Can you work these out from the model? Positions are in its coordinate system, mm. A direction names the side the tool comes from. Round coordinates to 2 decimals unless told otherwise and drop trailing zeros. Write each loop counter-clockwise with the first axis right and the second up, starting at its lowest first coordinate (ties: lowest second). Pieces come first, ordered by that corner, then holes. Notation, with made-up numbers: M 4,14 L 45,14 A4 ccw 45,19 Z; hole C -6,28.5 d4. An arc over 180 degrees is marked long. Answer as a JSON object with one key per item and string values. Group by question number.
1) I'm going to push flat-ended pins straight in: pin 1 Ø23 at (x, z) = (25.4, -25.4) entering from +Y; pin 2 Ø3 at (x, y) = (13, 72.5) entering from -Z; pin 3 Ø3 at (x, y) = (34.5, 38.5) entering from +Z. Where does each tip first touch, or does it pass through?
2) Suppose I cut it at D-D, the plane z = -990.6. Write out the boundary of the cut face in (x, y).
3) Suppose I cut it at B-B, the plane y = 104. Write out the boundary of the cut face in (x, z), and give its area (3 significant figures).
4) Suppose I cut it at C-C, the plane x = 25.4. State how many separate pieces and enclosed holes the cut face has, and give its area (3 significant figures).
5) Please list where these lines run through material, in increasing order: L1, parallel to Z at x = 25, y = 133; L2, parallel to Z at x = 27, y = 107; L3, parallel to Y at x = 44, z = -767.5. Write a range as [from, to].
6) Suppose I cut it at A-A, the plane z = -882. Write out the boundary of the cut face in (x, y), and give its area (3 significant figures).
7) On a 3-axis mill with a long thin cutter (end or side, diameter ignored), from which of +Z, -Z, +X, -X, +Y, -Y can I reach the whole of each face in a straight line? I mean faces 1 (the flat face through (26, 75, -76.2)), 2 (the flat face through (26, 13, -1016)), 3 (the flat face through (19, 127, -1002)), 4 (the flat face through (19, 127, -37)). Say none if no direction works.
8) If we mould it in two halves opening along Z, with no side actions, what happens to faces 5 (the cylindrical face through (23.747, 139.522, -978.008)), 6 (the flat face through (26, 0, -501)), 7 (the flat face through (25, 13, 0))? For each: +Z half, -Z half, draft (parallel to the pull), parting line (faces both ways), or undercut.
Autodesk Inventor part; units mm, degrees
ref_plane "YZ Plane" through (0, 0, 0) normal (1, 0, 0) x (0, 1, 0)
ref_plane "XZ Plane" through (0, 0, 0) normal (0, 1, 0) x (-1, 0, 0)
ref_plane "XY Plane" through (0, 0, 0) normal (0, 0, 1) x (1, 0, 0)
sketch "Sketch1" plane through (0, 0, 0) normal (0, 1, 0) x (-1, 0, 0)
  line L0 (0, 0) -> (-50.8, 0)
  line L1 (-50.8, 0) -> (-50.8, -1016)
  line L2 (-50.8, -1016) -> (0, -1016)
  line L3 (0, -1016) -> (0, 0)
  dimension "d0" = 1016
  dimension "d1" = 50.8
extrude "Extrusion1" add sketch "Sketch1" along normal blind 25.4
sketch "Sketch2" plane through (0, 25.4, 0) normal (0, 1, 0) x (1, 0, 0)
  line L0 (0, 50.8) -> (50.8, 50.8)
  line L1 (50.8, 50.8) -> (50.8, 76.2)
  line L2 (50.8, 76.2) -> (0, 76.2)
  line L3 (0, 76.2) -> (0, 50.8)
  line L4 (0, 965.2) -> (50.8, 965.2)
  line L5 (50.8, 965.2) -> (50.8, 939.8)
  line L6 (50.8, 939.8) -> (0, 939.8)
  line L7 (0, 939.8) -> (0, 965.2)
  line L8 (50.8, 1016) -> (0, 1016)
  line L9 (0, 0) -> (50.8, 0)
  dimension "d5" = 25.4
  dimension "d12" = 25.4
  dimension "d16" = 50.8
  dimension "d17" = 50.8
extrude "Extrusion2" add sketch "Sketch2" along normal blind 101.6
sketch "Sketch3" plane through (0, 25.4, 0) normal (0, 1, 0) x (1, 0, 0)
  circle A0 centre (25.4, 25.4) radius 12.7
  line L0 (0, 50.8) -> (0, 0)
  line L1 (0, 0) -> (50.8, 0)
  circle A1 centre (25.4, 990.6) radius 12.7
  line L2 (50.8, 1016) -> (0, 1016)
  line L3 (50.8, 965.2) -> (50.8, 1016)
  dimension "d18" = 25.4
  dimension "d19" = 25.4
  dimension "d20" = 25.4
  dimension "d21" = 25.4
  dimension "d22" = 25.4
  dimension "d23" = 25.4
sketch "Sketch4" plane through (0, 127, 0) normal (0, 1, 0) x (1, 0, 0)
  line L0 (0, 0) -> (50.8, 0)
  line L1 (50.8, 0) -> (50.8, 1016)
  line L2 (50.8, 1016) -> (0, 1016)
  line L3 (0, 1016) -> (0, 0)
extrude "Extrusion3" add sketch "Sketch4" along normal blind 25.4
extrude "Extrusion4" cut sketch "Sketch3" along normal blind 174.625 and the other way blind 63.5
properties part number "arm"
Results:
{
 "1": {"pin 1": "through", "pin 2": "z = -965.2", "pin 3": "z = -50.8"},
 "2": {"outline": "M 0,0 L 12.7,0 L 12.7,25.4 L 0,25.4 Z; M 0,127 L 12.7,127 L 12.7,152.4 L 0,152.4 Z; M 38.1,0 L 50.8,0 L 50.8,25.4 L 38.1,25.4 Z; M 38.1,127 L 50.8,127 L 50.8,152.4 L 38.1,152.4 Z"},
 "3": {"outline": "M 0,-965.2 L 50.8,-965.2 L 50.8,-939.8 L 0,-939.8 Z; M 0,-76.2 L 50.8,-76.2 L 50.8,-50.8 L 0,-50.8 Z", "area": "2,580 mm^2"},
 "4": {"separate pieces": "5", "enclosed holes": "1", "area": "54,200 mm^2"},
 "5": {"L1": "[-1016, -1003.29], [-977.91, -38.09], [-12.71, 0]", "L2": "[-965.2, -939.8], [-76.2, -50.8]", "L3": "[0, 25.4], [127, 152.4]"},
 "6": {"outline": "M 0,0 L 50.8,0 L 50.8,25.4 L 0,25.4 Z; M 0,127 L 50.8,127 L 50.8,152.4 L 0,152.4 Z", "area": "2,580 mm^2"},
 "7": {"face 1": "+X, -X", "face 2": "-Z, +X, -X, +Y, -Y", "face 3": "-Z, +X, -X", "face 4": "+Z, +X, -X"},
 "8": {"face 5": "undercut", "face 6": "draft", "face 7": "+Z half"}
}
